For this review, take the finished solid that the model builds, in its own axes (mm). Round coordinates to 2 decimals unless told otherwise and drop trailing zeros. Order: outer loops, then holes, each group sorted by start corner. A loop starts at its lowest first (then second) coordinate and runs counter-clockwise, first axis right, second up. Notation, with made-up numbers: (61, 11) -> (91, 11) arc R32 ccw to (91, 47) -> close; hole circle Ø10 at (61, -19.5). An arc over 180 degrees is marked (long way). Answer in a Markdown table with one row per item.
```python
from build123d import *

# Parameters (mm, degrees)
SKETCH1_W           = 25
SKETCH1_H           = 25
BOSS_EXTRUDE1_DEPTH = 25
SKETCH2_R           = 5.3
CUT_EXTRUDE1_DEPTH  = 38.5
FILLET1_RADIUS      = 12.5
FILLET1_LENGTH      = 25


with BuildPart() as part:
    # Sketch1 → Boss-Extrude1 (new body)
    with BuildSketch(Plane(origin=(0, 0, 0), x_dir=(1, 0, 0), z_dir=(0, 1, 0))):
        Rectangle(SKETCH1_W, SKETCH1_H)
    extrude(amount=BOSS_EXTRUDE1_DEPTH)

    # Sketch2 → Cut-Extrude1 (cut, through all)
    with BuildSketch(Plane.XY.offset(12.5)):
        with Locations((0, 12.5)):
            Circle(SKETCH2_R)
    extrude(amount=-CUT_EXTRUDE1_DEPTH, mode=Mode.SUBTRACT)

    # Fillet1: full round fillet: the end face becomes a half cylinder, R = half its width
    fillet1_face = Plane((0, 0, 0), x_dir=(0, 0, -1), z_dir=(0, -1, 0))  # on the end face: x along it, z out of the body
    fillet1_slab = fillet1_face.offset(-FILLET1_RADIUS / 2) * Box(FILLET1_LENGTH, 2 * FILLET1_RADIUS, FILLET1_RADIUS, mode=Mode.PRIVATE)  # the body's end, R deep
    fillet1_round = Plane((0, 12.5, 0), x_dir=(0, -1, 0), z_dir=(0, 0, -1)) * Cylinder(FILLET1_RADIUS, FILLET1_LENGTH, mode=Mode.PRIVATE)  # its axis R under the face
    add(fillet1_slab - fillet1_round, mode=Mode.SUBTRACT)


solid = part.part
```
Q1. Clearance check with flat-ended pins moving along their axes: pin 1 Ø1 at (y, z) = (9, 5.5) entering from -X; pin 2 Ø8 at (y, z) = (8, -6.5) entering from -X; pin 3 Ø5 at (y, z) = (8, -2) entering from -X. State where each tip first meets the part, or that it passes through.
Answer key:
| item | result |
|---|---|
| pin 1 | stops at x = -12.13 |
| pin 2 | stops at x = -12.49 |
| pin 3 | stops at x = -12.34 |
Q2. Take a section at A-A, the plane x = -4.75. Write out the cut boundary in (y, z), then the cut area to 3 significant figures.
Answer key:
| item | result |
|---|---|
| outline | (0.94, -12.5) -> (10.15, -12.5) -> (10.15, 12.5) -> (0.94, 12.5) -> close; (14.85, -12.5) -> (25, -12.5) -> (25, 12.5) -> (14.85, 12.5) -> close |
| area | 484 mm^2 |
Q3. Take a section at C-C, the plane y = 15. Write out the cut boundary in (x, z), then the cut area to 3 significant figures.
Answer key:
| item | result |
|---|---|
| outline | (-12.5, -12.5) -> (-4.67, -12.5) -> (-4.67, 12.5) -> (-12.5, 12.5) -> close; (4.67, -12.5) -> (12.5, -12.5) -> (12.5, 12.5) -> (4.67, 12.5) -> close |
| area | 391 mm^2 |
Q4. Take a section at D-D, the plane y = 2.5. Write out the cut boundary in (x, z).
Answer key:
| item | result |
|---|---|
| outline | (-7.5, -12.5) -> (7.5, -12.5) -> (7.5, 12.5) -> (-7.5, 12.5) -> close |
Q5. The part is to be moulded in two halves that separate along Y. For faces 1 (the face through (0, 18, -12.5)), 2 (the face through (-1.149, 7.326, 0.175)), 3 (the face through (0, 0, 0)), say which applies: +Y half, -Y half, draft (parallel to the pull), parting line (faces both ways), or undercut.
Answer key:
| item | result |
|---|---|
| face 1 | draft |
| face 2 | undercut |
| face 3 | -Y half |
Q6. To check wall thickness, follow probe 1 along Y at (x, z) = (0, 3.25); probe 2 along X at (y, z) = (14.5, 5.5); probe 3 along X at (y, z) = (15.5, -1). State the ranges of each line that lie inside material, in increasing order.
Answer key:
| item | result |
|---|---|
| probe 1 | y = 0 to 7.2, 17.8 to 25 |
| probe 2 | x = -12.5 to -4.91, 4.91 to 12.5 |
| probe 3 | x = -12.5 to -4.37, 4.37 to 12.5 |
Q7. Take a section at B-B, the plane z = -10.25. Write out the cut boundary in (x, y).
Answer key:
| item | result |
|---|---|
| outline | (-12.5, 12.5) arc R12.5 ccw to (12.5, 12.5) -> (12.5, 25) -> (-12.5, 25) -> close; hole circle Ø10.6 at (0, 12.5) |
